Check sheet for the modelled part. Datum: model origin and axes. Units: mm. Face numbers are marked on the shaded views. Round coordinates to 2 decimals unless told otherwise and drop trailing zeros. Write each loop counter-clockwise with the first axis right and the second up, starting at its lowest first coordinate (ties: lowest second). Pieces come first, ordered by that corner, then holes. Notation, with made-up numbers: (-33.5, 69.25) -> (-16.5, 69.25) arc R8 cw to (-16.5, 74.25) -> close; hole circle Ø4 at (6.5, -37.75). An arc over 180 degrees is marked (long way). Write item = value, one per line.
Autodesk Inventor part; units mm, degrees
ref_plane "YZ Plane" through (0, 0, 0) normal (1, 0, 0) x (0, 1, 0)
ref_plane "XZ Plane" through (0, 0, 0) normal (0, 1, 0) x (-1, 0, 0)
ref_plane "XY Plane" through (0, 0, 0) normal (0, 0, 1) x (1, 0, 0)
sketch "Sketch1" plane through (0, 0, 0) normal (0, 0, 1) x (1, 0, 0)
  line L0 (20, 8.5409) -> (80, 8.5409)
  line L1 (100, -11.4591) -> (100, -21.4591)
  line L2 (80, -41.4591) -> (20, -41.4591)
  line L3 (0, -21.4591) -> (0, -11.4591)
  arc A0 (20, 8.5409) -> (0, -11.4591) centre (20, -11.4591) ccw
  arc A1 (100, -11.4591) -> (80, 8.5409) centre (80, -11.4591) ccw
  arc A2 (80, -41.4591) -> (100, -21.4591) centre (80, -21.4591) ccw
  arc A3 (0, -21.4591) -> (20, -41.4591) centre (20, -21.4591) ccw
  point P0 (0, 0)
  point P1 (100, -41.4591)
  point P2 (100, 8.5409)
  point P3 (0, -41.4591)
  dimension "d0" = 100
  dimension "d1" = 50
  dimension "d2" = 20
extrude "Extrusion1" add sketch "Sketch1" along normal blind 40
sketch "Sketch3" plane through (0, 0, 40) normal (0, 0, 1) x (1, 0, 0)
  line L0 (26.6816, 5.0495) -> (71.4417, 5.0495)
  line L1 (71.4417, 5.0495) -> (71.4417, 1.6832)
  line L2 (71.4417, 1.6832) -> (26.6816, 1.6832)
  line L3 (26.6816, 1.6832) -> (26.6816, 5.0495)
  point P0 (0, 0)
extrude "Extrusion2" cut sketch "Sketch3" against normal blind 40
sketch "Sketch4" plane through (0, 0, 40) normal (0, 0, 1) x (1, 0, 0)
  circle A0 centre (35.5822, -15.1611) radius 7.5
  circle A1 centre (55.8486, -15.1611) radius 7.5
  point P0 (0, 0)
  dimension "d16" = 15
  dimension "d17" = 15
hole "Hole2" at (35.5822, -15.1611, 40) at (55.8486, -15.1611, 40) direction (0, 0, -1) diameter 15 end through all
properties part number "head"
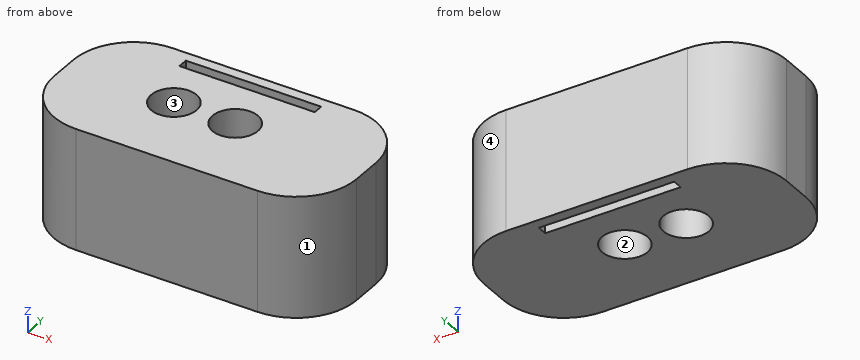
(1) Sectioned sample at D-D on z = 36.5. Enter the section's corners in (x, y).
Worked answers:
outline = (0, -21.46) arc R20 ccw to (20, -41.46) -> (80, -41.46) arc R20 ccw to (100, -21.46) -> (100, -11.46) arc R20 ccw to (80, 8.54) -> (20, 8.54) arc R20 ccw to (0, -11.46) -> close; hole (26.68, 1.68) -> (71.44, 1.68) -> (71.44, 5.05) -> (26.68, 5.05) -> close; hole circle Ø15 at (35.58, -15.16); hole circle Ø15 at (55.85, -15.16)
(2) Release check for a two-part mould opening along Y. For the marked faces 1, 2, 3 and 4 record: pulls with the +Y half, pulls with the -Y half, needs draft (parallel to the pull), parting line crosses it, or undercut.
Worked answers:
face_1 = pulls with the -Y half
face_2 = undercut
face_3 = undercut
face_4 = pulls with the +Y half
(3) Sectioned sample at C-C on x = 59.5. Enter the section's corners in (y, z), then the cut area to 3 significant figures.
Worked answers:
outline = (-41.46, 0) -> (-21.71, 0) -> (-21.71, 40) -> (-41.46, 40) -> close; (-8.61, 0) -> (1.68, 0) -> (1.68, 40) -> (-8.61, 40) -> close; (5.05, 0) -> (8.54, 0) -> (8.54, 40) -> (5.05, 40) -> close
area = 1,340 mm²
(4) Sectioned sample at A-A on x = 45.5. Enter the section's corners in (y, z).
Worked answers:
outline = (-41.46, 0) -> (1.68, 0) -> (1.68, 40) -> (-41.46, 40) -> close; (5.05, 0) -> (8.54, 0) -> (8.54, 40) -> (5.05, 40) -> close
(5) Sectioned sample at B-B on y = -20.5. Enter the section's corners in (x, z).
Worked answers:
outline = (0, 0) -> (30.31, 0) -> (30.31, 40) -> (0, 40) -> close; (40.85, 0) -> (50.58, 0) -> (50.58, 40) -> (40.85, 40) -> close; (61.12, 0) -> (100, 0) -> (100, 40) -> (61.12, 40) -> close
(6) Material ranges on L1, parallel to Y at x = 66.5, z = 29; L2, parallel to X at y = -12, z = 38.5; L3, parallel to X at y = -16, z = 21.5, recorded low to high. Write a range as [from, to].
Worked answers:
L1 = [-41.46, 1.68], [5.05, 8.54]
L2 = [0, 28.78], [42.38, 49.05], [62.65, 100]
L3 = [0, 28.13], [43.04, 48.4], [63.3, 100]
(7) Go/stop test with flat-tipped pins: P1, Ø5, axis at y = -0.5, z = 17, coming from the +X side; P2, Ø4, axis at y = -25, z = 13, coming from the +X side; P3, Ø3.5, axis at y = 3.5, z = 28, coming from the +X side. Record where each tip stops, or that it passes through.
Worked answers:
P1 = 98.12
P2 = 99.94
P3 = 95.02
